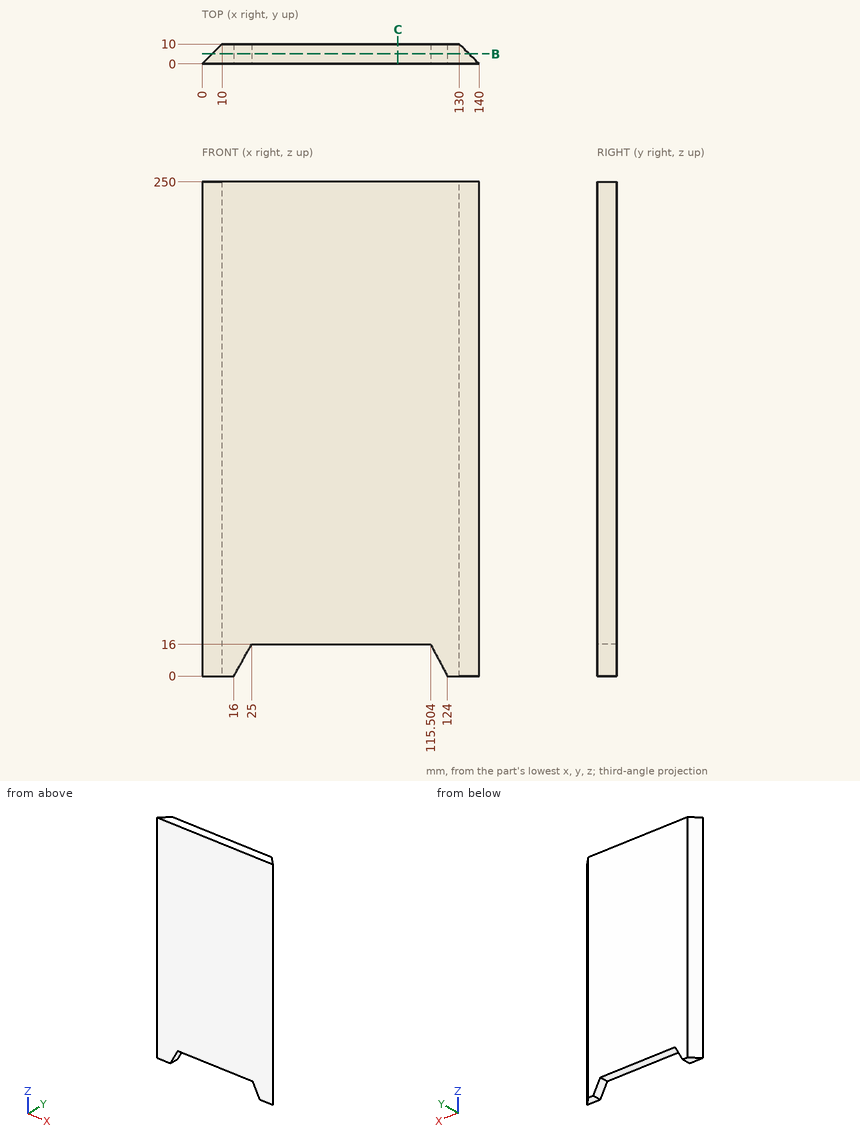
Input: dimensioned drawing with shaded views. Units: mm. Origin: part minimum x, y, z. Give positions to 0.01 mm unless a question says otherwise; leave off trailing zeros. Write each loop counter-clockwise with the first axis right and the second up, starting at its lowest first coordinate (ties: lowest second). Pieces come first, ordered by that corner, then holes. Notation, with made-up numbers: M 27,-33 L 32,-33 A26 ccw 32,-7 Z; hole C 89.5,51 d4. An arc over 180 degrees is marked long. Return JSON: item names as keys, results as strings. Group by question number.
1) Pin query (flat end, axial travel): P1, Ø1, axis at y = 1.5, z = 125.5, coming from the -X side; P2, Ø3, axis at x = 61, y = 4.5, coming from the -Z side. Return the tip coordinate at first contact, or that it passes through.
2) Cut plane C-C, the plane x = 99. Output: boundary loops of the cut face in (y, z), plus the area to 3 significant figures.
3) Cut plane B-B, the plane y = 5. Output: boundary loops of the cut face in (x, z), plus the area to 3 significant figures.
4) Material intervals for line 1 along Z through (x, y) = (40, 8); line 2 along X through (y, z) = (0.5, 153.5); line 3 along X through (y, z) = (1.75, 195.5), sorted ascending. Write a range as [from, to].
Recorded:
{
 "1": {"P1": "stops at x = 1", "P2": "stops at z = 16"},
 "2": {"outline": "M 0,16 L 10,16 L 10,250 L 0,250 Z", "area": "2,340 mm²"},
 "3": {"outline": "M 5,0 L 16,0 L 25,16 L 115.5,16 L 124,0 L 135,0 L 135,250 L 5,250 Z", "area": "30,900 mm²"},
 "4": {"line 1": "z = [16, 250]", "line 2": "x = [0.5, 139.5]", "line 3": "x = [1.75, 138.25]"}
}
